Design review of the part built by this model. Coordinates are the model's own, in mm. Face numbers are marked on the shaded views. A direction names the side the tool comes from. Round coordinates to 2 decimals unless told otherwise and drop trailing zeros. Loops run counter-clockwise (first coordinate to the right, second up) from the corner with the lowest first, then second, coordinate; pieces in that order, holes last. Notation, with made-up numbers: (88, 29) - (145, 29) arc R9 cw to (145, 42) - close; hole circle Ø11 at (38, 51). An arc over 180 degrees is marked (long way). Return JSON: item names as keys, results as strings. Group by question number.
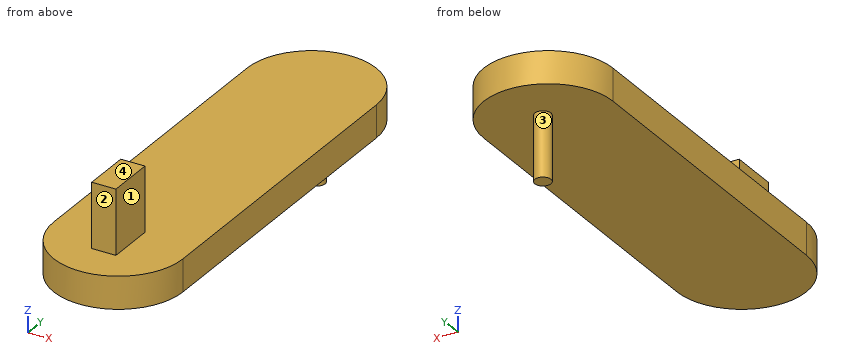
from build123d import *

# Parameters (mm, degrees)
F1_DEPTH = 50.8
F2_R     = 12.7
F3_DEPTH = 101.6
F4_W     = 38.1
F4_H     = 76.2
F5_DEPTH = 101.6


with BuildPart() as f1:
    # F0 (on Top) → F1 (new body)
    with BuildSketch(Plane.XY):
        with BuildLine():
            Line((-101.6, 508), (-101.6, 0))
            ThreePointArc((-101.6, 0), (0, -101.6), (101.6, 0))
            Line((101.6, 0), (101.6, 508))
            ThreePointArc((101.6, 508), (0, 609.6), (-101.6, 508))
        make_face()
    extrude(amount=-F1_DEPTH)

    # F2 (on face) → F3 (join)
    with BuildSketch(Plane(origin=(0, 0, -50.8), x_dir=(1, 0, 0), z_dir=(0, 0, -1))):
        with Locations((0, -522.219658)):
            Circle(F2_R)
    extrude(amount=F3_DEPTH)

    # F4 (on face) → F5 (join)
    with BuildSketch(Plane.XY):
        Rectangle(F4_W, F4_H)
    extrude(amount=F5_DEPTH)


solid = f1.part
Q1. Tool access review of the marked faces 1, 2, 3 and 4: name each direction out of +Z, -Z, +X, -X, +Y, -Y from which nothing blocks a thin tool from reaching the whole face with its end or side.
Q2. Add section D-D, the plane z = -88. State the section outline as (x, y) points, plus the area to 3 significant figures.
Q3. Add section C-C, the plane y = 188.5. State the section outline as (x, z) points, plus the area to 3 significant figures.
Q4. For line 1 (Z direction, x = 55.5, y = 269.5); line 2 (Z direction, x = 13, y = -23); line 3 (X direction, y = 26.5, z = 44.5), list the stretches that pass through material, from the lowest coordinate up.
Q5. Insertion check: pin 1 Ø1.5 at (x, y) = (-36.5, 126) entering from -Z; pin 2 Ø23 at (y, z) = (-17, 62.5) entering from -X; pin 3 Ø8 at (x, z) = (-15.5, -101.5) entering from +Y. Each pin has a flat end and moves straight along its axis. Give the tip position at first contact, or say it passes through.
Q6. Add section B-B, the plane z = 52. State the section outline as (x, y) points, plus the area to 3 significant figures.
Q7. Add section A-A, the plane x = 0. State the section outline as (y, z) points, plus the area to 3 significant figures.
Evaluation:
{
 "1": {"face 1": "+Z, +X, +Y, -Y", "face 2": "+Z, +X, -X, -Y", "face 3": "-Z", "face 4": "+Z, +X, -X, +Y, -Y"},
 "2": {"outline": "circle Ø25.4 at (0, 522.22)", "area": "507 mm²"},
 "3": {"outline": "(-101.6, -50.8) - (101.6, -50.8) - (101.6, 0) - (-101.6, 0) - close", "area": "10,300 mm²"},
 "4": {"line 1": "-50.8 to 0", "line 2": "-50.8 to 101.6", "line 3": "-19.05 to 19.05"},
 "5": {"pin 1": "z = -50.8", "pin 2": "x = -19.05", "pin 3": "y = 527.61"},
 "6": {"outline": "(-19.05, -38.1) - (19.05, -38.1) - (19.05, 38.1) - (-19.05, 38.1) - close", "area": "2,900 mm²"},
 "7": {"outline": "(-101.6, -50.8) - (509.52, -50.8) - (509.52, -152.4) - (534.92, -152.4) - (534.92, -50.8) - (609.6, -50.8) - (609.6, 0) - (38.1, 0) - (38.1, 101.6) - (-38.1, 101.6) - (-38.1, 0) - (-101.6, 0) - close", "area": "46,500 mm²"}
}
